```python
from build123d import *

# Parameters (mm, degrees)
SKETCH1_W           = 156.9
SKETCH1_H           = 65.6
BOSS_EXTRUDE1_DEPTH = 2.6
SKETCH2_W           = 7
SKETCH2_H           = 2.6
BOSS_EXTRUDE2_DEPTH = 7
SKETCH3_R           = 1.49999999
CUT_EXTRUDE1_DEPTH  = 103.712815656
FILLET1_R           = 5
CUT_EXTRUDE2_DEPTH  = 3.5
FILLET3_R           = 5
CHAMFER1_SIZE       = 0.25


with BuildPart() as part:
    # Sketch1 → Boss-Extrude1 (new body)
    with BuildSketch(Plane(origin=(0, 0, 0), x_dir=(1, 0, 0), z_dir=(0, 1, 0))):
        Rectangle(SKETCH1_W, SKETCH1_H)
    extrude(amount=BOSS_EXTRUDE1_DEPTH)

    # Sketch2 → Boss-Extrude2 (add)
    with BuildSketch(Plane(origin=(0, 2.6, 0), x_dir=(1, 0, 0), z_dir=(0, 1, 0))):
        with Locations((-74.95, 31.5)):
            Rectangle(SKETCH2_W, SKETCH2_H)
        with Locations((-74.95, -31.5)):
            Rectangle(SKETCH2_W, SKETCH2_H)
        with Locations((74.95, -31.5)):
            Rectangle(SKETCH2_W, SKETCH2_H)
        with Locations((74.95, 31.5)):
            Rectangle(SKETCH2_W, SKETCH2_H)
    extrude(amount=BOSS_EXTRUDE2_DEPTH)

    # Sketch3 → Cut-Extrude1 (cut, through all)
    with BuildSketch(Plane(origin=(0, 0, -32.8), x_dir=(-1, 0, 0), z_dir=(0, 0, -1))):
        with BuildLine():
            Line((-78.45, 9.6), (-78.45, 6.1))
            ThreePointArc((-78.45, 6.1), (-77.424873734, 8.574873734), (-74.95, 9.6))
            Line((-74.95, 9.6), (-78.45, 9.6))
        make_face()
        with BuildLine():
            Line((-71.45, 9.6), (-74.95, 9.6))
            ThreePointArc((-74.95, 9.6), (-72.475126266, 8.574873734), (-71.45, 6.1))
            Line((-71.45, 6.1), (-71.45, 9.6))
        make_face()
        with Locations((74.95, 6.1)):
            Circle(SKETCH3_R)
        with BuildLine():
            Line((74.95, 9.6), (71.45, 9.6))
            Line((71.45, 9.6), (71.45, 6.1))
            ThreePointArc((71.45, 6.1), (72.475126266, 8.574873734), (74.95, 9.6))
        make_face()
        with BuildLine():
            Line((78.45, 9.6), (74.95, 9.6))
            ThreePointArc((74.95, 9.6), (77.424873734, 8.574873734), (78.45, 6.1))
            Line((78.45, 6.1), (78.45, 9.6))
        make_face()
        with Locations((-74.95, 6.1)):
            Circle(SKETCH3_R)
    extrude(amount=-CUT_EXTRUDE1_DEPTH, mode=Mode.SUBTRACT)

    # Fillet1
    # the kernel refuses this fillet: 5 mm, written as the material it adds along each edge
    with BuildSketch(Plane(origin=(-71.45, 2.6, 32.8), x_dir=(1, 0, 0), z_dir=(0, 0, -1))) as fillet1_piece_1:
        with BuildLine():
            CenterArc((4.866600265, -5), FILLET1_R, 90, 79.835751378)
            Line((-0.054929303, -4.117647059), (-0.547082259, -4.029411765))
            ThreePointArc((-0.547082259, -4.029411765), (-0.5, -3.5), (-0.5, 0))
            Line((-0.5, 0), (0, 0.5))
            Line((0, 0.5), (4.866600265, 0.5))
            Line((4.866600265, 0.5), (4.866600265, 0))
        make_face()
    extrude(amount=2.6)
    with BuildSketch(Plane(origin=(71.45, 2.6, 32.8), x_dir=(0.01333878666755776, 0.9999110344276821, 0), z_dir=(0, 0, -1)), Plane(origin=(-71.45, 2.6, -32.8), x_dir=(-0.013338786667550865, 0.9999110344276821, 0), z_dir=(0, 0, 1))) as fillet1_piece_2:
        with BuildLine():
            CenterArc((4.934640629, -4.932861239), FILLET1_R, 99.399969777, 79.835751378)
            Line((-0.064914543, -4.866167305), (-0.56487006, -4.859497912))
            Line((-0.56487006, -4.859497912), (-0.499955517, 0.006669393))
            Line((-0.499955517, 0.006669393), (0.006669393, 0.499955517))
            ThreePointArc((0.006669393, 0.499955517), (3.506358014, 0.453269764), (4.036350699, 0.493286124))
            Line((4.036350699, 0.493286124), (4.11801342, 0))
        make_face()
    extrude(amount=2.6)
    with BuildSketch(Plane(origin=(71.45, 2.6, -32.8), x_dir=(0.01333878666755776, 0.9999110344276821, 0), z_dir=(0, 0, 1))) as fillet1_piece_3:
        with BuildLine():
            CenterArc((4.934640629, 4.932861239), FILLET1_R, 180.764278845, 79.835751378)
            Line((-0.064914543, 4.866167305), (-0.56487006, 4.859497912))
            Line((-0.56487006, 4.859497912), (-0.499955517, -0.006669393))
            Line((-0.499955517, -0.006669393), (0.006669393, -0.499955517))
            ThreePointArc((0.006669393, -0.499955517), (3.506358014, -0.453269764), (4.036350699, -0.493286124))
            Line((4.036350699, -0.493286124), (4.11801342, 0))
        make_face()
    extrude(amount=2.6)

    # Sketch4 → Cut-Extrude2 (cut)
    with BuildSketch(Plane(origin=(0, 2.6, 0), x_dir=(1, 0, 0), z_dir=(0, 1, 0))):
        Polygon((-62.45, -24.8), (0, -2.707525213), (62.45, -24.8), align=None)
        Polygon((-66.45, -20.8), (-66.45, 20.8), (-7.653508772, 0), align=None)
        Polygon((66.45, -20.8), (66.45, 20.8), (7.653508772, 0), align=None)
        Polygon((-62.45, 24.8), (62.45, 24.8), (0, 2.707525213), align=None)
    extrude(amount=-CUT_EXTRUDE2_DEPTH, mode=Mode.SUBTRACT)

    # Fillet3
    fillet3_edges = [part.edges().sort_by_distance(p)[0] for p in [
        (0, 1.3, -2.707525213),
        (-62.45, 1.3, -24.8),
        (62.45, 1.3, -24.8),
        (-7.653508772, 1.3, 0),
        (-66.45, 1.3, 20.8),
        (-66.45, 1.3, -20.8),
        (66.45, 1.3, 20.8),
        (7.653508772, 1.3, 0),
        (66.45, 1.3, -20.8),
        (62.45, 1.3, 24.8),
        (-62.45, 1.3, 24.8),
        (0, 1.3, 2.707525213),
    ]]
    fillet(fillet3_edges, radius=FILLET3_R)

    # Chamfer1
    chamfer1_edges = [part.edges().sort_by_distance(p)[0] for p in [
        (-73.45000001, 6.1, -30.2),
        (-73.45000001, 6.1, 30.2),
        (76.44999999, 6.1, 30.2),
        (76.44999999, 6.1, -30.2),
    ]]
    chamfer(chamfer1_edges, length=CHAMFER1_SIZE)


solid = part.part
```
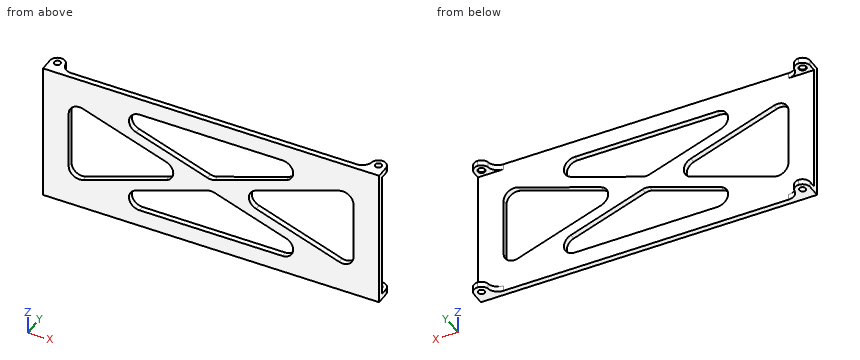
Build history of the part. All positions in model axes, mm. Coordinates: 2 decimals unless noted, no trailing zeros. Order: outer loops, then holes, each group sorted by start corner. A loop starts at its lowest first (then second) coordinate and runs counter-clockwise, first axis right, second up.
Item 1: Drop flat-ended pins along their axis: pin 1 Ø5 at (x, y) = (74.95, 6.1) entering from -Z; pin 2 Ø19.5 at (x, z) = (-23.5, 5) entering from +Y. Give the stop position or say it passes through.
Filled in:
pin 1: stops at z = -32.8
pin 2: stops at y = 2.6
Item 2: Drill centre lines: L1, parallel to Z at x = -19, y = 0.75; L2, parallel to Y at x = -74.95, z = -31.8; L3, parallel to Z at x = -1, y = 0.5. Where is each one in solid material? Low to high.
Filled in:
L1: z = -32.8 to -24.8, -9.43 to -3.42, 3.42 to 9.43, 24.8 to 32.8
L2: y = 0 to 4.6, 7.6 to 9.6
L3: z = -32.8 to -24.8, -3.11 to 3.11, 24.8 to 32.8
Item 3: Saw through at B-B on z = 23. List the corners of the cut face in (x, y).
Filled in:
outline: (-78.45, 0) - (-37.17, 0) - (-37.17, 2.6) - (-78.45, 2.6) - close; (37.17, 0) - (78.45, 0) - (78.45, 2.6) - (37.17, 2.6) - close
Item 4: Saw through at D-D on z = -28. List the corners of the cut face in (x, y), then the cut area to 3 significant figures.
Filled in:
outline: (-78.45, 0) - (78.45, 0) - (78.45, 2.6) - (-78.45, 2.6) - close
area: 408 mm2
Item 5: Saw through at C-C on x = -14.5. List the corners of the cut face in (y, z), then the cut area to 3 significant figures.
Filled in:
outline: (0, -32.8) - (2.6, -32.8) - (2.6, -24.8) - (0, -24.8) - close; (0, -7.84) - (2.6, -7.84) - (2.6, 7.84) - (0, 7.84) - close; (0, 24.8) - (2.6, 24.8) - (2.6, 32.8) - (0, 32.8) - close
area: 82.4 mm2
Item 6: Saw through at A-A on x = -56. List the corners of the cut face in (y, z), then the cut area to 3 significant figures.
Filled in:
outline: (0, -32.8) - (2.6, -32.8) - (2.6, -17.1) - (0, -17.1) - close; (0, 17.1) - (2.6, 17.1) - (2.6, 32.8) - (0, 32.8) - close
area: 81.6 mm2
